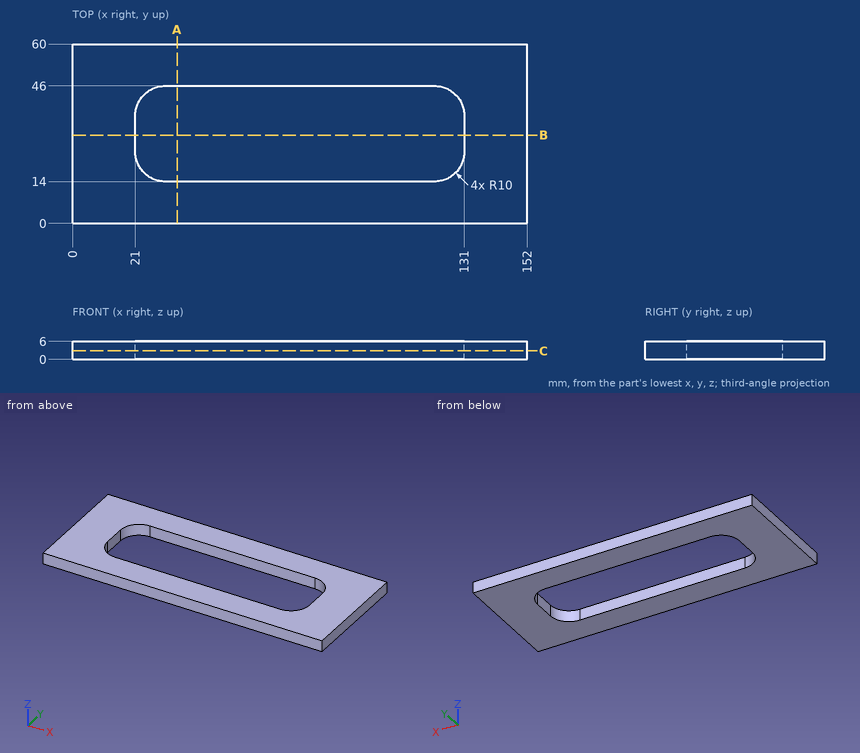
Could you check a few things on this drawing? It's one solid part, dimensions in mm from its lowest x, y, z. Coordinates: 2 decimals unless noted, no trailing zeros. Write each loop counter-clockwise with the first axis right and the second up, starting at its lowest first coordinate (ties: lowest second). Pieces come first, ordered by that corner, then holes. Notation, with made-up numbers: (-25, 47) - (-6, 47) arc R31 ccw to (-6, 86) - close; hole circle Ø7 at (41, 67). An arc over 180 degrees is marked (long way). Put each result on its own line as item: value. Start each with the question number.
Q1. I want a section at C-C on z = 2.85. Write out the boundary of the cut face in (x, y), plus the area to 3 significant figures.
Q2. Please list where these lines run through material, in increasing order: L1, parallel to Y at x = 89, z = 5.75; L2, parallel to X at y = 23.5, z = 2.85; L3, parallel to X at y = 40.5, z = 5.5.
Q3. I want a section at A-A on x = 35. Write out the boundary of the cut face in (y, z).
Q4. I want a section at B-B on y = 29.5. Write out the boundary of the cut face in (x, z), plus the area to 3 significant figures.
Checks:
1. outline: (0, 0) - (152, 0) - (152, 60) - (0, 60) - close; hole (21, 24) arc R10 ccw to (31, 14) - (121, 14) arc R10 ccw to (131, 24) - (131, 36) arc R10 ccw to (121, 46) - (31, 46) arc R10 ccw to (21, 36) - close
1. area: 5,690 mm²
2. L1: 0 to 14, 46 to 60
2. L2: 0 to 21.01, 130.99 to 152
2. L3: 0 to 22.07, 129.93 to 152
3. outline: (0, 0) - (14, 0) - (14, 6) - (0, 6) - close; (46, 0) - (60, 0) - (60, 6) - (46, 6) - close
4. outline: (0, 0) - (21, 0) - (21, 6) - (0, 6) - close; (131, 0) - (152, 0) - (152, 6) - (131, 6) - close
4. area: 252 mm²
